```python
from build123d import *

# Parameters (mm, degrees)
SKETCH_2_R          = 1.5
CUT_EXTRUDE_1_DEPTH = 28.820855486


with BuildPart() as part:
    # Эскиз1 → Повернуть1 (revolve)
    with BuildSketch(Plane.XY, mode=Mode.PRIVATE) as revolve_1_sk:
        Polygon((0, 4), (0, 7), (2, 7), (2, 15), (8, 15), (8, 7), (20, 7), (20, 4), align=None)
    revolve(revolve_1_sk.sketch.rotate(Axis((8, 0, 0), (-1, 0, 0)), 90), axis=Axis((8, 0, 0), (-1, 0, 0)))

    # Эскиз2 → Вырез-Вытянуть1 (cut, through all)
    with BuildSketch(Plane.ZY.offset(-2)):
        with Locations((0, 11)):
            Circle(SKETCH_2_R)
        with Locations((-11, 0)):
            Circle(SKETCH_2_R)
        with Locations((0, -11)):
            Circle(SKETCH_2_R)
        with Locations((11, 0)):
            Circle(SKETCH_2_R)
    extrude(amount=-CUT_EXTRUDE_1_DEPTH, mode=Mode.SUBTRACT)


solid = part.part
```
Can you work these out from the model? Positions are in its coordinate system, mm. A direction names the side the tool comes from. Give positions to 0.01 mm unless a question says otherwise; leave off trailing zeros. Loops run counter-clockwise (first coordinate to the right, second up) from the corner with the lowest first, then second, coordinate; pieces in that order, holes last. Notation, with made-up numbers: M 26.25,46 L 39.25,46 A7 cw 39.25,55 Z; hole C 9.25,-19 d7. An arc over 180 degrees is marked long. Use CSV: the item, a comma, the result in double quotes. Start each with the question number.
1. Imagine slicing it at A-A, the plane y = 0. Write out the boundary of the cut face in (x, z), plus the area to 3 significant figures.
2. If we mould it in two halves opening along Z, with no side actions, what happens to faces 1 (the face through (4.96, 0.07, 9.5)), 2 (the face through (14.08, 6.21, -3.23)), 3 (the face through (20, 3, -3))? For each: released by +Z, released by -Z, zero draft, split by the parting line, or undercut.
3. Imagine slicing it at C-C, the plane x = 7.25. Write out the boundary of the cut face in (y, z).
4. On a 3-axis mill with a long thin cutter (end or side, diameter ignored), from which of +Z, -Z, +X, -X, +Y, -Y can I reach the whole of each face in a straight line? I mean faces 4 (the face through (0, 3, 3)), 5 (the face through (2, 3.1, 6.5)), 6 (the face through (8, 6.5, -3.1)). Say none if no direction works.
5. Imagine slicing it at D-D, the plane z = -11. Write out the boundary of the cut face in (x, y).
6. If I drill on L1, parallel to Y at x = 3.3, z = 0; L2, parallel to X at y = 10, z = 7.25; L3, parallel to Y at x = 7.75, z = -1, over which ranges is the centre line in solid material (lowest first)?
7. For P1, Ø10, axis at x = 7, y = -6.5, coming from the +Z side; P2, Ø6, axis at x = 2, z = 11.5, coming from the -Y side; P3, Ø1, axis at y = 5.5, z = -5.5, coming from the +X side, each with a flat end and sliding along its axis, tell me the tip position at first contact or that it passes through.
Response values:
1,outline,"M 0,-7 L 2,-7 L 2,-9.5 L 8,-9.5 L 8,-7 L 20,-7 L 20,-4 L 0,-4 Z; M 0,4 L 20,4 L 20,7 L 8,7 L 8,9.5 L 2,9.5 L 2,7 L 0,7 Z; M 2,-15 L 8,-15 L 8,-12.5 L 2,-12.5 Z; M 2,12.5 L 8,12.5 L 8,15 L 2,15 Z"
1,area,"180 mm^2"
2,face 1,"undercut"
2,face 2,"split by the parting line"
2,face 3,"zero draft"
3,outline,"C 0,0 d30; hole C -11,0 d3; hole C 0,0 d8; hole C 0,-11 d3; hole C 0,11 d3; hole C 11,0 d3"
4,face 4,"+Z, -Z, -X, +Y, -Y"
4,face 5,"-X"
4,face 6,"+X"
5,outline,"M 2,-10.2 L 8,-10.2 L 8,-1.5 L 2,-1.5 Z; M 2,1.5 L 8,1.5 L 8,10.2 L 2,10.2 Z"
6,L1,"-15 to -12.5, -9.5 to -4, 4 to 9.5, 12.5 to 15"
6,L2,"2 to 8"
6,L3,"-14.97 to -12.12, -9.88 to -3.87, 3.87 to 9.88, 12.12 to 14.97"
7,P1,"z = 14.92"
7,P2,"y = -12.36"
7,P3,"x = 8"
